Autodesk Inventor part; units mm, degrees
ref_plane "工作平面1" through (0, 0, 3) normal (0, 0, 1) x (1, 0, 0)
ref_plane "工作平面2" through (25.5, -42.8342, 3) normal (0.5115346, -0.8592627, 0) x (0.8592627, 0.5115346, 0)
ref_plane "工作平面3" through (-25.5, -42.8342, 3) normal (-0.5115346, -0.8592627, 0) x (0.8592627, -0.5115346, 0)
sketch "草圖1" plane through (0, 0, 0) normal (0, 0, 1) x (1, 0, 0)
  circle A0 centre (0, 0) radius 49.85
  circle A1 centre (0, 0) radius 43
  dimension "d0" = 99.7
  dimension "d3" = 86
extrude "擠出1" add sketch "草圖1" along normal blind 6
sketch "草圖2" plane through (0, 0, 6) normal (0, 0, 1) x (1, 0, 0)
  circle A0 centre (0, 0) radius 43
  circle A1 centre (0, 0) radius 49.85
  line L0 (0, 0) -> (0, 49.85)
  line L1 (11, 48.6212) -> (11, 41.5692)
  line L2 (-11, 48.6212) -> (-11, 41.5692)
  dimension "d6" = 22
extrude "擠出2" cut sketch "草圖2" against normal blind 4 contours A0 L0 A1 L1 | L2 A1 L0 A0
ref_plane "工作平面1" through (0, 0, 3) normal (0, 0, 1) x (1, 0, 0)
sketch "草圖3" plane through (0, 0, 3) normal (0, 0, 1) x (1, 0, 0)
  line L0 (0, 0) -> (0, -42.4806)
  line L1 (0, 0) -> (-25.5, -42.8342)
  line L2 (0, 0) -> (25.5, -42.8342)
  arc A0 (-11, 48.6212) -> (11, 48.6212) centre (0, 0) ccw
  line L3 (-25.5, -42.8342) -> (25.5, -42.8342)
  dimension "d9" = 51
  dimension "d27" = 61.532
  dimension "d28" = 30.766
  dimension "d29" = 30.766
ref_plane "工作平面2" through (25.5, -42.8342, 3) normal (0.5115346, -0.8592627, 0) x (0.8592627, 0.5115346, 0)
ref_plane "工作平面3" through (-25.5, -42.8342, 3) normal (-0.5115346, -0.8592627, 0) x (0.8592627, -0.5115346, 0)
sketch "草圖4" plane through (25.5, -42.8342, 3) normal (0.5115346, -0.8592627, 0) x (0.8592627, 0.5115346, 0)
  point P0 (0, -3)
  point P1 (0, 0)
hole "孔1" at (25.5, -42.8342, 3) direction (-0.5115346, 0.8592627, 0) diameter 3 depth 2.5 tip angle 118
sketch "草圖5" plane through (-25.5, -42.8342, 3) normal (-0.5115346, -0.8592627, 0) x (0.8592627, -0.5115346, 0)
  point P0 (0, -3)
  point P1 (0, 0)
hole "孔2" at (-25.5, -42.8342, 3) direction (0.5115346, 0.8592627, 0) diameter 3 depth 2.5 tip angle 118
chamfer "倒角1" distance 0.5 angle 45 5 edges at (-26.2298, -34.0735, 6) (34.0735, 26.2298, 6) (-49.85, 0, 0) (-31.1181, -38.9447, 6) (38.9447, 31.1181, 6)
properties part number "KE-SP-02-P1"
Read the model definition and answer for the solid it produces. Units are mm, in the model's axes. A direction names the side the tool comes from. Give positions to 0.01 mm unless a question says otherwise; leave off trailing zeros. Loops run counter-clockwise (first coordinate to the right, second up) from the corner with the lowest first, then second, coordinate; pieces in that order, holes last. Notation, with made-up numbers: (38, -1) - (82, -1) arc R24 ccw to (82, 10) - close; hole circle Ø9 at (-40, -12.5). An arc over 180 degrees is marked (long way). Answer as CSV lines item,"result". Start each with the question number.
1) Find section B-B (x = 0). Write down the section's boundary in (y, z), then the cut area to 3 significant figures.
2) Straight lines are drawn through the part: L1, parallel to X at y = 0, z = 1.35; L2, parallel to X at y = 35, z = 2.5; L3, parallel to Y at x = 0, z = 2.4. For each, find the intervals that lie inside material, in ascending order. Write a range as from..to.
3) Each of these flat-tipped pins is pushed along its axis until it touches: pin 1 Ø1.2 at (y, z) = (46, 4) entering from +X; pin 2 Ø1.5 at (x, z) = (17, 4) entering from -Y; pin 3 Ø9 at (x, y) = (-4, 46) entering from +Z. Where does it stop, or does it pass through?
4) Which of the six approach directions +Z, -Z, +X, -X, +Y, -Y give full straight-line access (tool end or side, diameter ignored) to faces 4 (the face through (23.907, -40.006, 2.752)), 5 (the face through (11, 45, 4)), 6 (the face through (-6.489, -49.426, 2.965))?
5) Find section A-A (y = 0). Write down the section's boundary in (x, z), then the cut area to 4 significant figures.
6) Determine the mould class of faces 1 (the face through (-23.926, -39.995, 2.759)), 2 (the face through (2.02, -49.45, 5.86)), 3 (the face through (3, 44, 0)) for opening direction Z: released by +Z, released by -Z, zero draft, split by the parting line, or undercut.
Findings below:
1,outline,"(-49.85, 0.5) - (-49.35, 0) - (-43, 0) - (-43, 5.5) - (-43.5, 6) - (-49.35, 6) - (-49.85, 5.5) - close; (43, 0) - (49.35, 0) - (49.85, 0.5) - (49.85, 2) - (43, 2) - close"
1,area,"54.3 mm^2"
2,L1,"-49.85..-43, 43..49.85"
2,L2,"-35.5..-24.98, 24.98..35.5"
2,L3,"-49.85..-43"
3,pin 1,"x = 20.59"
3,pin 2,"y = -47.13"
3,pin 3,"z = 2"
4,face 4,"none"
4,face 5,"+Z, +Y"
4,face 6,"+Z, -Z"
5,outline,"(-49.85, 0.5) - (-49.35, 0) - (-43, 0) - (-43, 5.5) - (-43.5, 6) - (-49.35, 6) - (-49.85, 5.5) - close; (43, 0) - (49.35, 0) - (49.85, 0.5) - (49.85, 5.5) - (49.35, 6) - (43.5, 6) - (43, 5.5) - close"
5,area,"81.45 mm^2"
6,face 1,"undercut"
6,face 2,"released by +Z"
6,face 3,"released by -Z"
